Autodesk Inventor part; units mm, degrees
ref_plane "side_4d_XY" through (-20, 0, -330) normal (-1, 0, 0) x (0, 1, 0)
ref_plane "side_4d_YZ" through (-20, 0, -330) normal (0, 1, 0) x (0, 0, -1)
ref_plane "side_4d_ZX" through (-20, 0, -330) normal (0, 0, -1) x (-1, 0, 0)
sketch "Skizze_1" plane through (0, 0, 0) normal (0, 0, 1) x (1, 0, 0)
  arc A0 (-20, -17) -> (-17, -20) centre (-17, -17) ccw
  line L0 (-17, -20) -> (-4.1, -20)
  line L1 (-4.1, -20) -> (-4.1, -17)
  line L2 (-4.1, -17) -> (-10.5, -17)
  line L3 (-10.5, -17) -> (-10.5, -13.6627)
  arc A1 (-10.0314, -12.5314) -> (-10.5, -13.6627) centre (-8.9002, -13.6627) ccw
  line L4 (-10.0314, -12.5314) -> (-7.4645, -9.9645)
  arc A2 (-3.9289, -8.5) -> (-7.4645, -9.9645) centre (-3.9289, -13.5) ccw
  line L5 (-3.9289, -8.5) -> (3.9289, -8.5)
  arc A3 (7.4645, -9.9645) -> (3.9289, -8.5) centre (3.9289, -13.5) ccw
  line L6 (7.4645, -9.9645) -> (10.0314, -12.5314)
  arc A4 (10.5, -13.6627) -> (10.0314, -12.5314) centre (8.9002, -13.6627) ccw
  line L7 (10.5, -13.6627) -> (10.5, -17)
  line L8 (10.5, -17) -> (4.1, -17)
  line L9 (4.1, -17) -> (4.1, -20)
  line L10 (4.1, -20) -> (17, -20)
  arc A5 (17, -20) -> (20, -17) centre (17, -17) ccw
  line L11 (20, -17) -> (20, -4.1)
  line L12 (20, -4.1) -> (17, -4.1)
  line L13 (17, -4.1) -> (17, -10.5)
  line L14 (17, -10.5) -> (13.6627, -10.5)
  arc A6 (12.5314, -10.0314) -> (13.6627, -10.5) centre (13.6627, -8.9002) ccw
  line L15 (12.5314, -10.0314) -> (9.9645, -7.4645)
  arc A7 (8.5, -3.9289) -> (9.9645, -7.4645) centre (13.5, -3.9289) ccw
  line L16 (8.5, -3.9289) -> (8.5, 3.9289)
  arc A8 (9.9645, 7.4645) -> (8.5, 3.9289) centre (13.5, 3.9289) ccw
  line L17 (9.9645, 7.4645) -> (12.5314, 10.0314)
  arc A9 (13.6627, 10.5) -> (12.5314, 10.0314) centre (13.6627, 8.9002) ccw
  line L18 (13.6627, 10.5) -> (17, 10.5)
  line L19 (17, 10.5) -> (17, 4.1)
  line L20 (17, 4.1) -> (20, 4.1)
  line L21 (20, 4.1) -> (20, 17)
  arc A10 (20, 17) -> (17, 20) centre (17, 17) ccw
  line L22 (17, 20) -> (4.1, 20)
  line L23 (4.1, 20) -> (4.1, 17)
  line L24 (4.1, 17) -> (10.5, 17)
  line L25 (10.5, 17) -> (10.5, 13.6627)
  arc A11 (10.0314, 12.5314) -> (10.5, 13.6627) centre (8.9002, 13.6627) ccw
  line L26 (10.0314, 12.5314) -> (7.4645, 9.9645)
  arc A12 (3.9289, 8.5) -> (7.4645, 9.9645) centre (3.9289, 13.5) ccw
  line L27 (3.9289, 8.5) -> (-3.9289, 8.5)
  arc A13 (-7.4645, 9.9645) -> (-3.9289, 8.5) centre (-3.9289, 13.5) ccw
  line L28 (-7.4645, 9.9645) -> (-10.0314, 12.5314)
  arc A14 (-10.5, 13.6627) -> (-10.0314, 12.5314) centre (-8.9002, 13.6627) ccw
  line L29 (-10.5, 13.6627) -> (-10.5, 17)
  line L30 (-10.5, 17) -> (-4.1, 17)
  line L31 (-4.1, 17) -> (-4.1, 20)
  line L32 (-4.1, 20) -> (-17, 20)
  arc A15 (-17, 20) -> (-20, 17) centre (-17, 17) ccw
  line L33 (-20, 17) -> (-20, 4.1)
  line L34 (-20, 4.1) -> (-17, 4.1)
  line L35 (-17, 4.1) -> (-17, 10.5)
  line L36 (-17, 10.5) -> (-13.6627, 10.5)
  arc A16 (-12.5314, 10.0314) -> (-13.6627, 10.5) centre (-13.6627, 8.9002) ccw
  line L37 (-12.5314, 10.0314) -> (-9.9645, 7.4645)
  arc A17 (-8.5, 3.9289) -> (-9.9645, 7.4645) centre (-13.5, 3.9289) ccw
  line L38 (-8.5, 3.9289) -> (-8.5, -3.9289)
  arc A18 (-9.9645, -7.4645) -> (-8.5, -3.9289) centre (-13.5, -3.9289) ccw
  line L39 (-9.9645, -7.4645) -> (-12.5314, -10.0314)
  arc A19 (-13.6627, -10.5) -> (-12.5314, -10.0314) centre (-13.6627, -8.9002) ccw
  line L40 (-13.6627, -10.5) -> (-17, -10.5)
  line L41 (-17, -10.5) -> (-17, -4.1)
  line L42 (-17, -4.1) -> (-20, -4.1)
  line L43 (-20, -4.1) -> (-20, -17)
  circle A20 centre (0, 0) radius 6
extrude "Extrusion1" add sketch "Skizze_1" along normal blind 720
sketch "Sketch2" plane through (0, 0, 0) normal (0, 0, -1) x (1, 0, 0)
  point P0 (-15, -15)
hole "Drilling 1" at (-15, 15, 0) direction (0, 0, 1) diameter 5 depth 6000
sketch "Sketch3" plane through (0, 0, 0) normal (0, 0, -1) x (1, 0, 0)
  point P0 (15, -15)
hole "Drilling 2" at (15, 15, 0) direction (0, 0, 1) diameter 5 depth 6000
sketch "Sketch4" plane through (0, 0, 0) normal (0, 0, -1) x (1, 0, 0)
  point P0 (15, 15)
hole "Drilling 3" at (15, -15, 0) direction (0, 0, 1) diameter 5 depth 6000
sketch "Sketch5" plane through (0, 0, 0) normal (0, 0, -1) x (1, 0, 0)
  point P0 (-15, 15)
hole "Drilling 4" at (-15, -15, 0) direction (0, 0, 1) diameter 5 depth 6000
ref_plane "side_4d_XY" through (-20, 0, -330) normal (-1, 0, 0) x (0, 1, 0)
ref_plane "side_4d_YZ" through (-20, 0, -330) normal (0, 1, 0) x (0, 0, -1)
ref_plane "side_4d_ZX" through (-20, 0, -330) normal (0, 0, -1) x (-1, 0, 0)
ref_plane "side_1a_XY" through (0, 20, -330) normal (0, 1, 0) x (1, 0, 0)
ref_plane "side_1a_YZ" through (0, 20, -330) normal (1, 0, 0) x (0, 0, -1)
ref_plane "side_1a_ZX" through (0, 20, -330) normal (0, 0, -1) x (0, 1, 0)
ref_plane "side_2b_XY" through (20, 0, -330) normal (1, 0, 0) x (0, -1, 0)
ref_plane "side_2b_YZ" through (20, 0, -330) normal (0, -1, 0) x (0, 0, -1)
ref_plane "side_2b_ZX" through (20, 0, -330) normal (0, 0, -1) x (1, 0, 0)
ref_plane "side_3c_XY" through (0, -20, -330) normal (0, -1, 0) x (-1, 0, 0)
ref_plane "side_3c_YZ" through (0, -20, -330) normal (-1, 0, 0) x (0, 0, -1)
ref_plane "side_3c_ZX" through (0, -20, -330) normal (0, 0, -1) x (0, -1, 0)
ref_plane "end_XY" through (0, 0, -660) normal (0, 0, -1) x (1, 0, 0)
ref_plane "end_YZ" through (0, 0, -660) normal (1, 0, 0) x (0, -1, 0)
ref_plane "end_ZX" through (0, 0, -660) normal (0, -1, 0) x (0, 0, -1)
ref_plane "start_XY" through (0, 0, 0) normal (0, 0, 1) x (1, 0, 0)
ref_plane "start_YZ" through (0, 0, 0) normal (1, 0, 0) x (0, 1, 0)
ref_plane "start_ZX" through (0, 0, 0) normal (0, 1, 0) x (0, 0, 1)
properties part number "MayTec 1.11.040040.43S_Profile 40x40, 4E, S_660_Detail_(0;0,0,0)"
Design review of the part built by this model. Coordinates are the model's own, in mm. Give positions to 0.01 mm unless a question says otherwise; leave off trailing zeros. Use a Markdown table: item, result. Add a question column.
(1) Add section A-A on z = 630. Give the number of separate pieces and of enclosed holes in the cut face, then the cut area to 3 significant figures.
(2) Mouldability with a two-part tool opening along X and no side actions: class faces 1 (the face through (-6, 0, 355)), 2 (the face through (-20, -10, 355)), 3 (the face through (10, -20, 355)), 4 (the face through (20, 10, 355)) as +X half, -X half, draft (parallel to the pull), parting line (faces both ways), or undercut.
(3) Wall thickness on probe 1 along X at (y, z) = (15, 384); probe 2 along X at (y, z) = (-16.5, 166.5): over which ranges is each line inside the solid? List them lowest first. Write a range as [from, to].
(4) Clearance check with flat-ended pins moving along their axes: P1, Ø4, axis at x = 15, y = -15, coming from the -Z side; P2, Ø5, axis at x = -0.5, z = 633.5, coming from the +Y side; P3, Ø3.5, axis at x = -19, z = 480, coming from the -Y side; P4, Ø2, axis at y = 1.5, z = 514.5, coming from the -X side. State where each tip first meets the part, or that it passes through.
Report:
| question | item | result |
|---|---|---|
| 1 | separate pieces | 1 |
| 1 | enclosed holes | 5 |
| 1 | area | 674 mm² |
| 2 | face 1 | undercut |
| 2 | face 2 | -X half |
| 2 | face 3 | draft |
| 2 | face 4 | +X half |
| 3 | probe 1 | x = [-20, -17.5], [-12.5, -10.5], [10.5, 12.5], [17.5, 20] |
| 3 | probe 2 | x = [-20, -17], [-13, -10.5], [10.5, 13], [17, 20] |
| 4 | P1 | passes through |
| 4 | P2 | stops at y = 8.5 |
| 4 | P3 | stops at y = -19.99 |
| 4 | P4 | stops at x = -8.5 |
